For this review, take the finished solid that the model builds, in its own axes (mm). Face numbers are marked on the shaded views. A direction names the side the tool comes from. Give positions to 0.01 mm unless a question says otherwise; leave off trailing zeros. Loops run counter-clockwise (first coordinate to the right, second up) from the corner with the lowest first, then second, coordinate; pieces in that order, holes last.
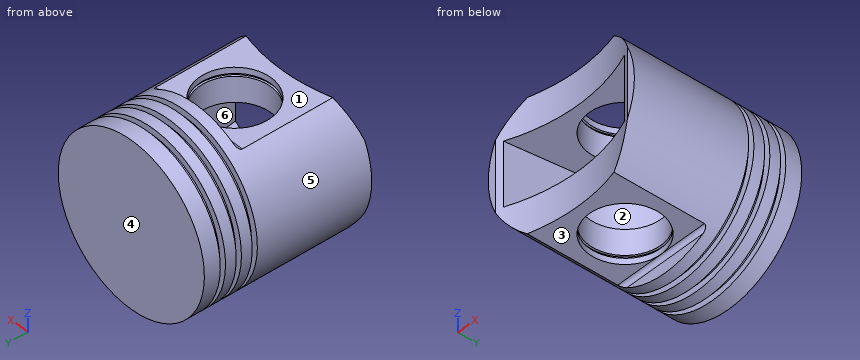
```python
from build123d import *

# Parameters (mm, degrees)
SKETCH_13_R              = 41
EXTRUDE_3_DEPTH          = 42
CUT_EXTRUDE_1_DEPTH      = 72.596089278675
CUT_EXTRUDE_1_DEPTH_BACK = 72.596089278675
SKETCH_14_R              = 17.999999999999996
CUT_EXTRUDE_START        = -52
CUT_EXTRUDE_3_DEPTH      = 52
CUT_EXTRUDE_4_DEPTH      = 16
CUT_EXTRUDE_START_2      = -8
SKETCH_20_R              = 41
SKETCH_20_R_2            = 37.8
CUT_EXTRUDE_5_DEPTH      = 2.6
PATTERN_LINEAR_1_COUNT   = 3
PATTERN_LINEAR_1_PITCH   = 8
FILLET_1_R               = 2


with BuildPart() as part:
    # Эскиз13 → Бобышка-Вытянуть3 (new, symmetric)
    with BuildSketch(Plane(origin=(0, 0, 0), x_dir=(1, 0, 0), z_dir=(0, 1, 0))):
        with Locations(Location((0, 0, 0), (0, 0, 90))):
            Circle(SKETCH_13_R)
    extrude(amount=EXTRUDE_3_DEPTH, both=True)

    # Эскиз14 → Вырез-Вытянуть1 (cut, two sides: drawn at the far end of the back side and taken through both)
    with BuildSketch(Plane.XY.offset(-CUT_EXTRUDE_1_DEPTH_BACK)):
        with BuildLine():
            Line((-37.09447398198258, -41.99999999999993), (37.09447398198258, -41.99999999999993))
            ThreePointArc((37.09447398198258, -41.99999999999993), (5.51e-15, -34.00000000000003), (-37.09447398198258, -41.99999999999993))
        make_face()
        with Locations((0, -10.000000000000009)):
            Circle(SKETCH_14_R)
    extrude(amount=CUT_EXTRUDE_1_DEPTH + CUT_EXTRUDE_1_DEPTH_BACK, mode=Mode.SUBTRACT)

    # Эскиз16 → Вырез-Вытянуть3 (cut)
    with BuildSketch(Plane.XZ.offset(42).offset(CUT_EXTRUDE_START)):
        with BuildLine():
            ThreePointArc((24.331050121192877, 33), (2.51e-15, 41), (-24.33105012119288, 33))
            Line((-24.331050121192874, 33), (24.331050121192874, 33))
        make_face()
        with BuildLine():
            Line((24.331050121192874, -33), (-24.331050121192874, -33))
            ThreePointArc((-24.331050121192902, -32.99999999999998), (-7.53e-15, -41), (24.331050121192863, -33.000000000000014))
        make_face()
    extrude(amount=CUT_EXTRUDE_3_DEPTH, mode=Mode.SUBTRACT)

    # Эскиз18 → Вырез-Вытянуть4 (cut, symmetric)
    with BuildSketch(Plane.XY):
        with BuildLine():
            Line((-29.77638454923953, -6.3439196978451875), (-34.154400712657626, -42.00000000000001))
            Line((-34.154400712657626, -42.00000000000001), (34.15440071265802, -42.00000000000002))
            Line((34.15440071265802, -42.00000000000002), (29.7763845492392, -6.3439196978452435))
            ThreePointArc((29.7763845492392, -6.3439196978452435), (1.516e-14, 19.999999999999574), (-29.77638454923953, -6.3439196978451875))
        make_face()
    extrude(amount=CUT_EXTRUDE_4_DEPTH, both=True, mode=Mode.SUBTRACT)

    # Эскиз20 → Вырез-Вытянуть5 (cut)
    with BuildSketch(Plane(origin=(0, 42, 0), x_dir=(1, 0, 0), z_dir=(0, 1, 0)).offset(CUT_EXTRUDE_START_2)):
        with Locations(Location((0, 0, 0), (0, 0, 53.598479946))):
            Circle(SKETCH_20_R)
        with Locations(Location((0, 0, 0), (0, 0, 270))):
            Circle(SKETCH_20_R_2, mode=Mode.SUBTRACT)
    cut_extrude_5 = extrude(amount=-CUT_EXTRUDE_5_DEPTH, mode=Mode.SUBTRACT)

    # Линейный массив1: Вырез-Вытянуть5 ×3
    with Locations(*[(0, -i * PATTERN_LINEAR_1_PITCH, 0) for i in range(1, PATTERN_LINEAR_1_COUNT)]):
        add(cut_extrude_5, mode=Mode.SUBTRACT)

    # Скругление1
    fillet_1_edges = [part.edges().sort_by_distance(p)[0] for p in [
        (0, 10, 33),
        (0, 10, -33),
    ]]
    fillet(fillet_1_edges, radius=FILLET_1_R)

    # Эскиз24 → Вырез-Повернуть3 (revolve, cut)
    with BuildSketch(Plane(origin=(0, 0, 0), x_dir=(0, 0, -1), z_dir=(1, 0, 0)), mode=Mode.PRIVATE) as cut_revolve_3_sk:
        Polygon((-30.000000000000085, -29.00000000000005), (-28.600000000000087, -29.000000000000053), (-28.60000000000009, -10.000000000000053), (-30.000000000000085, -10.000000000000053), align=None)
        Polygon((28.600000000000215, -10.000000000000046), (28.600000000000218, -29.000000000000046), (30.000000000000213, -29.000000000000043), (30.00000000000021, -10.000000000000046), align=None)
    revolve(cut_revolve_3_sk.sketch.rotate(Axis((0, -10.000000000000009, -456.95829419610067), (0, 0, 1)), 90), axis=Axis((0, -10.000000000000009, -456.95829419610067), (0, 0, 1)), mode=Mode.SUBTRACT)


solid = part.part
```
Q1. Mouldability with a two-part tool opening along X and no side actions: class the marked faces 4, 5 and 6 as +X half, -X half, draft (parallel to the pull), parting line (faces both ways), or undercut.
Answers:
face 4: draft
face 5: parting line
face 6: undercut
Q2. Consider section C-C on y = 13.5. Give the boundary of the cut face in (x, z).
Answers:
outline: circle Ø82 at (0, 0); hole (-18.65, -16) - (18.65, -16) - (18.65, 16) - (-18.65, 16) - close
Q3. Machinability: for the marked faces 1, 2 and 3, which of the approach directions +Z, -Z, +X, -X, +Y, -Y give a long, thin tool a straight path to every point of the face, cutting with its end or side? Answer none if there is none.
Answers:
face 1: +Z, +X, -X, -Y
face 2: -Y
face 3: -Z, +X, -X, -Y
Q4. For pin 1 Ø3 at (x, y) = (-17, 3) entering from +Z; pin 2 Ø19 at (x, y) = (-2, -5) entering from +Z; pin 3 Ø2 at (y, z) = (-12.5, -10.5) entering from -X; pin 4 Ø1.8 at (x, z) = (1, -37) entering from -Y, all flat-tipped, find the tip position at first contact; note any pin that passes through.
Answers:
pin 1: stops at z = 33
pin 2: passes through
pin 3: stops at x = -39.88
pin 4: stops at y = 10
Q5. For probe 1 along Y at (x, z) = (15, -36); probe 2 along Y at (x, z) = (0, -31); probe 3 along Y at (x, z) = (0, 29.2), list the stretches that pass through material, from the lowest coordinate up.
Answers:
probe 1: y = 10 to 15.4, 18 to 23.4, 26 to 31.4, 34 to 42
probe 2: y = -34 to -28, 8 to 42
probe 3: y = -34 to -29, 9 to 42
